Verification items for the finished model (mm, model axes). Face numbers are marked on the shaded views. A direction names the side the tool comes from. Round coordinates to 2 decimals unless told otherwise and drop trailing zeros. Loops run counter-clockwise (first coordinate to the right, second up) from the corner with the lowest first, then second, coordinate; pieces in that order, holes last.
from build123d import *

# Parameters (mm, degrees)
SKETCH_1_R      = 3.95
EXTRUDE_1_DEPTH = 2.3
SKETCH_2_R      = 1.85
EXTRUDE_2_DEPTH = 1.6
SKETCH_3_R      = 3.05
EXTRUDE_3_DEPTH = 3
DRAFT_7_ANGLE   = -20
FILLET_1_R      = 1


with BuildPart() as part:
    # 草图1 → 凸台-拉伸1 (new body)
    with BuildSketch(Plane.XY):
        Circle(SKETCH_1_R)
    extrude(amount=EXTRUDE_1_DEPTH)

    # 草图2 → 凸台-拉伸2 (add)
    with BuildSketch(Plane.XY.offset(2.3)):
        Circle(SKETCH_2_R)
    extrude(amount=EXTRUDE_2_DEPTH)

    # 草图3 → 凸台-拉伸3 (add)
    with BuildSketch(Plane.XY.offset(3.9)):
        Circle(SKETCH_3_R)
    extrude(amount=EXTRUDE_3_DEPTH)

    # 拔模7
    draft_7_faces = [part.faces().sort_by_distance(p)[0] for p in [
        (-3.05, 0, 5.4),
    ]]
    draft(draft_7_faces, Plane(origin=(0, 0, 3.9), x_dir=(-1, 0, 0), z_dir=(0, 0, -1)), DRAFT_7_ANGLE)

    # 圆角1
    fillet_1_edges = [part.edges().sort_by_distance(p)[0] for p in [
        (-3.95, 0, 0),
    ]]
    fillet(fillet_1_edges, radius=FILLET_1_R)


solid = part.part
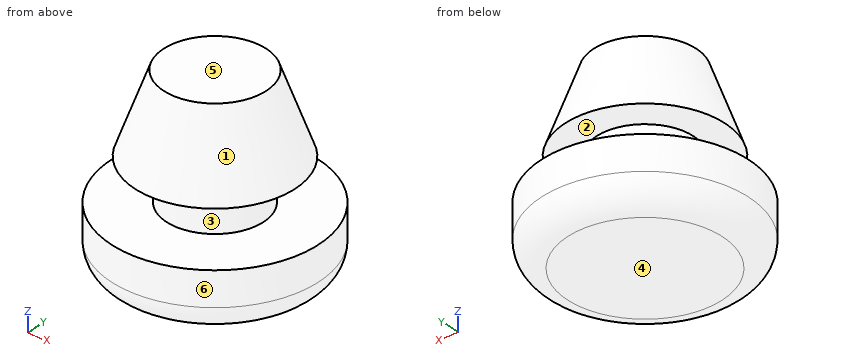
1. Section check D-D (z = 0.75). Enter the section's corners in (x, y).
2. Scan lines: L1, parallel to X at y = 1.5, z = 5.5; L2, parallel to Z at x = -1.5, y = 1.5; L3, parallel to Z at x = 3, y = 1.25. Record each from-to range of solid material in increasing order.
3. Section check A-A (y = 0). Enter the section's corners in (x, z), then the cut area to 3 significant figures.
4. Tool access check on the marked faces 1 and 2. Record the directions out of +Z, -Z, +X, -X, +Y, -Y that give a thin tool (end or side, any length) a straight path to the whole face; none if there is none.
5. Gauge pin test, flat end, axial feed: P1, Ø3, axis at x = -2.5, z = 5.5, coming from the -Y side. Record the tip position at first contact, or that the pin passes through.
6. Release check for a two-part mould opening along Z. For the marked faces 3, 4, 5 and 6 record: released by +Z, released by -Z, zero draft, split by the parting line, or undercut.
7. Section check C-C (z = 3). Enter the section's corners in (x, y).
Taken from the geometry:
1. outline: circle Ø7.84 at (0, 0)
2. L1: x = -1.96 to 1.96
2. L2: z = 0 to 2.3, 3.9 to 6.45
2. L3: z = 0.05 to 2.3
3. outline: (-3.95, 1) arc R1 ccw to (-2.95, 0) - (2.95, 0) arc R1 ccw to (3.95, 1) - (3.95, 2.3) - (1.85, 2.3) - (1.85, 3.9) - (3.05, 3.9) - (1.96, 6.9) - (-1.96, 6.9) - (-3.05, 3.9) - (-1.85, 3.9) - (-1.85, 2.3) - (-3.95, 2.3) - close
3. area: 38.7 mm2
4. face 1: +Z
4. face 2: none
5. P1: stops at y = -2.47
6. face 3: undercut
6. face 4: released by -Z
6. face 5: released by +Z
6. face 6: zero draft
7. outline: circle Ø3.7 at (0, 0)
